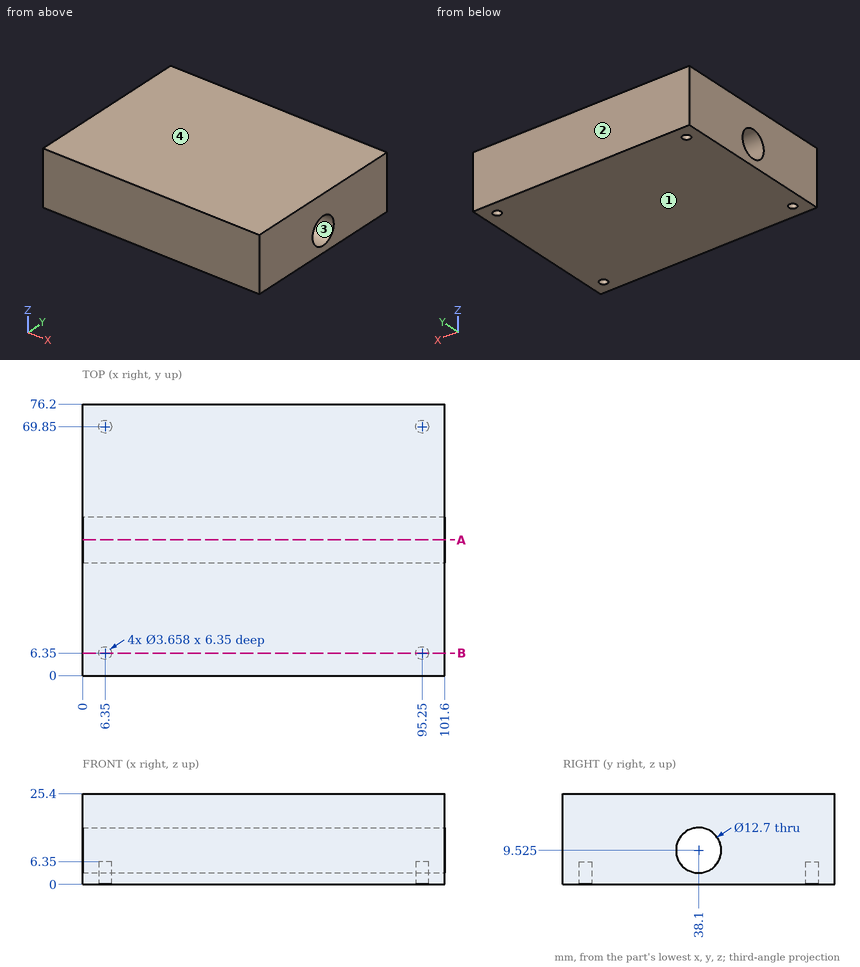
Geometry: see drawing. Coordinates: mm, zero at the bounding-box minimum. Round coordinates to 2 decimals unless told otherwise and drop trailing zeros. Loops run counter-clockwise (first coordinate to the right, second up) from the corner with the lowest first, then second, coordinate; pieces in that order, holes last. Notation, with made-up numbers: (-14, 45) - (45, 45) arc R30 ccw to (45, 73) - close; hole circle Ø2 at (-21, 3). An arc over 180 degrees is marked (long way). Write item = value, one per line. Start each with the question number.
(1) Pull-direction query (Z, two-part tool) for the marked faces 1, 2, 3 and 4; classes: +Z half, -Z half, draft (parallel to the pull), parting line (faces both ways), or undercut.
(2) Ray query, line 1 along X through (y, z) = (69.85, 2.5); line 2 along Y through (x, z) = (95.25, 2.5); line 3 along Y through (x, z) = (95.25, 4). Return the intervals inside material, ascending. Write a range as from..to.
(3) Section query B-B, the plane y = 6.35. Output: boundary loops of the cut face in (x, z).
(4) Pin query (flat end, axial travel): pin 1 (3 mm diameter, centred on x = 6.35, y = 69.85, fed in from -Z); pin 2 (10 mm diameter, centred on y = 38.1, z = 9.525, fed in from -X) (3 decimals). Return the tip coordinate at first contact, or that it passes through.
(5) Section query A-A, the plane y = 38.1. Output: boundary loops of the cut face in (x, z) (1 decimal), plus the area to 3 significant figures.
Conclusion:
q1.face_1 = -Z half
q1.face_2 = draft
q1.face_3 = undercut
q1.face_4 = +Z half
q2.line_1 = 0..4.52, 8.18..93.42, 97.08..101.6
q2.line_2 = 0..4.52, 8.18..68.02, 71.68..76.2
q2.line_3 = 0..4.52, 8.18..34.97, 41.23..68.02, 71.68..76.2
q3.outline = (0, 0) - (4.52, 0) - (4.52, 6.35) - (8.18, 6.35) - (8.18, 0) - (93.42, 0) - (93.42, 6.35) - (97.08, 6.35) - (97.08, 0) - (101.6, 0) - (101.6, 25.4) - (0, 25.4) - close
q4.pin_1 = 6.35
q4.pin_2 = through
q5.outline = (0, 0) - (101.6, 0) - (101.6, 3.2) - (0, 3.2) - close; (0, 15.9) - (101.6, 15.9) - (101.6, 25.4) - (0, 25.4) - close
q5.area = 1,290 mm2
